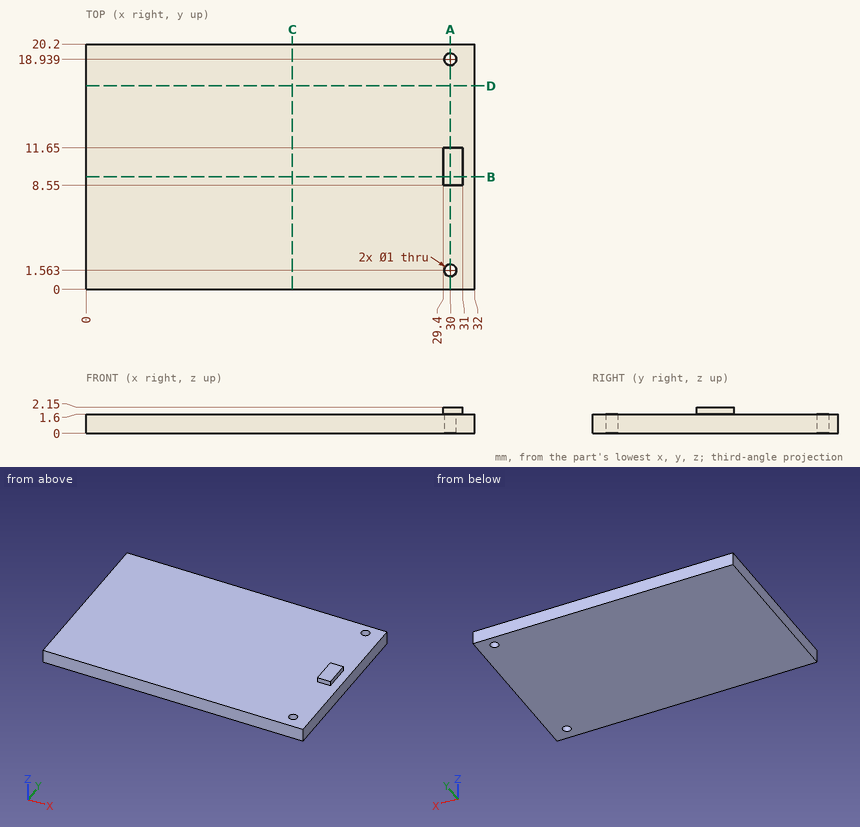
Geometry: see drawing. Coordinates: mm, zero at the bounding-box minimum. Round coordinates to 2 decimals unless told otherwise and drop trailing zeros. Order: outer loops, then holes, each group sorted by start corner. A loop starts at its lowest first (then second) coordinate and runs counter-clockwise, first axis right, second up. Notation, with made-up numbers: (0, 41) - (10, 41) arc R15 cw to (10, 51) - close; hole circle Ø8 at (10, 56). An arc over 180 degrees is marked (long way). One line per question, with ' | ' between items. Start each with the question number.
1) Cut plane C-C, the plane x = 17. Return the cut outline in (y, z).
2) Cut plane A-A, the plane x = 30. Return the cut outline in (y, z).
3) Cut plane D-D, the plane y = 16.75. Return the cut outline in (x, z).
4) Contact query for flat-ended pins moving along their axis: P1, Ø4, axis at x = 7.5, y = 14, coming from the +Z side; P2, Ø0.6, axis at y = 10, z = 2, coming from the +X side. Output: stop coordinate, or through.
5) Cut plane B-B, the plane y = 9.25. Return the cut outline in (x, z), then the cut area to 3 significant figures.
6) Ray query, probe 1 along Y at (x, z) = (30, 0.8); probe 2 along Z at (x, y) = (6, 4.5). Return the intervals inside material, ascending.
Worked out:
1) outline: (0, 0) - (20.2, 0) - (20.2, 1.6) - (0, 1.6) - close
2) outline: (0, 0) - (1.06, 0) - (1.06, 1.6) - (0, 1.6) - close; (2.06, 0) - (18.44, 0) - (18.44, 1.6) - (11.65, 1.6) - (11.65, 2.15) - (8.55, 2.15) - (8.55, 1.6) - (2.06, 1.6) - close; (19.44, 0) - (20.2, 0) - (20.2, 1.6) - (19.44, 1.6) - close
3) outline: (0, 0) - (32, 0) - (32, 1.6) - (0, 1.6) - close
4) P1: stops at z = 1.6 | P2: stops at x = 31
5) outline: (0, 0) - (32, 0) - (32, 1.6) - (31, 1.6) - (31, 2.15) - (29.4, 2.15) - (29.4, 1.6) - (0, 1.6) - close | area: 52.1 mm^2
6) probe 1: y = 0 to 1.06, 2.06 to 18.44, 19.44 to 20.2 | probe 2: z = 0 to 1.6
